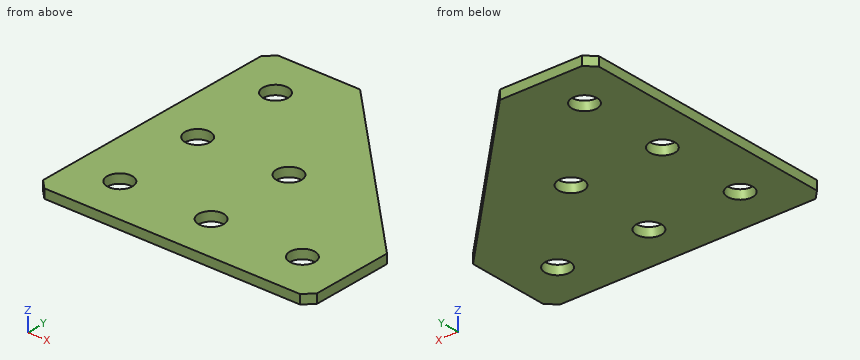
from build123d import *

# Parameters (mm, degrees)
EXTRUDE_1_DEPTH   = 2
HOLE_WIZARD_M51_D = 5.5
CHAMFER_1_SIZE    = 2


with BuildPart() as part:
    # Эскиз1 → Бобышка-Вытянуть1 (new body)
    with BuildSketch(Plane(origin=(0, 0, 0), x_dir=(1, 0, 0), z_dir=(0, 0, -1))):
        Polygon((0, 0), (0, 60), (60, 60), (60, 40), (20, 0), align=None)
    extrude(amount=EXTRUDE_1_DEPTH)

    # Отверстие с зазором M51 (through all)
    with Locations(Plane(origin=(0, 0, -2), x_dir=(1, 0, 0), z_dir=(0, 0, -1))):
        with Locations((30, 50), (10, 50), (10, 30), (10, 10), (50, 50), (30, 30)):
            Hole(HOLE_WIZARD_M51_D / 2)

    # Фаска1
    chamfer_1_edges = [part.edges().sort_by_distance(p)[0] for p in [
        (0, 0, -1),
        (0, -60, -1),
        (60, -60, -1),
    ]]
    chamfer(chamfer_1_edges, length=CHAMFER_1_SIZE)


solid = part.part
Model file for the job. Use its own axes, mm. Give positions to 0.01 mm unless a question says otherwise; leave off trailing zeros. Loops run counter-clockwise (first coordinate to the right, second up) from the corner with the lowest first, then second, coordinate; pieces in that order, holes last. Notation, with made-up numbers: (-2, 72.25) -> (38, 72.25) arc R35 cw to (38, 107.25) -> close; hole circle Ø7 at (55, 55.5). An arc over 180 degrees is marked (long way). Use a Markdown table: item, result. Add a question column.
(1) Slice it at D-D on x = 50. List the corners of the cut face in (y, z).
(2) Drop a flat-ended pin along its axis: pin 1 Ø1 at (y, z) = (-36, -0.5) entering from +X. Give the stop position or say it passes through.
(3) Slice it at A-A on x = 10. List the corners of the cut face in (y, z).
(4) Wall check: line 1 along X through (y, z) = (-50, -1.35); line 2 along Y through (x, z) = (10, -0.9); line 3 along Y through (x, z) = (11, -1.8). Give the ranges that are in metal, low to high.
(5) Slice it at B-B on y = -30. List the corners of the cut face in (x, z).
(6) Slice it at C-C on y = -10. List the corners of the cut face in (x, z), and give its area (3 significant figures).
Filled sheet:
| question | item | result |
|---|---|---|
| 1 | outline | (-60, -2) -> (-52.75, -2) -> (-52.75, 0) -> (-60, 0) -> close; (-47.25, -2) -> (-30, -2) -> (-30, 0) -> (-47.25, 0) -> close |
| 2 | pin 1 | x = 56.5 |
| 3 | outline | (-60, -2) -> (-52.75, -2) -> (-52.75, 0) -> (-60, 0) -> close; (-47.25, -2) -> (-32.75, -2) -> (-32.75, 0) -> (-47.25, 0) -> close; (-27.25, -2) -> (-12.75, -2) -> (-12.75, 0) -> (-27.25, 0) -> close; (-7.25, -2) -> (0, -2) -> (0, 0) -> (-7.25, 0) -> close |
| 4 | line 1 | 0 to 7.25, 12.75 to 27.25, 32.75 to 47.25, 52.75 to 60 |
| 4 | line 2 | -60 to -52.75, -47.25 to -32.75, -27.25 to -12.75, -7.25 to 0 |
| 4 | line 3 | -60 to -52.56, -47.44 to -32.56, -27.44 to -12.56, -7.44 to 0 |
| 5 | outline | (0, -2) -> (7.25, -2) -> (7.25, 0) -> (0, 0) -> close; (12.75, -2) -> (27.25, -2) -> (27.25, 0) -> (12.75, 0) -> close; (32.75, -2) -> (50, -2) -> (50, 0) -> (32.75, 0) -> close |
| 6 | outline | (0, -2) -> (7.25, -2) -> (7.25, 0) -> (0, 0) -> close; (12.75, -2) -> (30, -2) -> (30, 0) -> (12.75, 0) -> close |
| 6 | area | 49.0 mm2 |
